from build123d import *

# Parameters (mm, degrees)
SKETCH_1_R      = 4
SKETCH_1_R_2    = 2
EXTRUDE_1_DEPTH = 2.8
SKETCH_1_3_R    = 2
EXTRUDE_2_DEPTH = 25
FILLET_1_R      = 0.5


with BuildPart() as part:
    # Sketch 1 → Extrude 1 (new body)
    # profile 1 of 2: a face of its own
    with BuildSketch(Plane(origin=(0, 0, 0), x_dir=(1, 0, 0), z_dir=(0, 1, 0))):
        with Locations(Location((0, 0, 0), (0, 0, 270))):
            Circle(SKETCH_1_R)
        Circle(SKETCH_1_R_2, mode=Mode.SUBTRACT)
    # profile 2 of 2: a face of its own
    with BuildSketch(Plane(origin=(0, 0, 0), x_dir=(1, 0, 0), z_dir=(0, 1, 0))):
        Circle(SKETCH_1_R_2)
    extrude(amount=EXTRUDE_1_DEPTH)

    # Sketch 1_3 → Extrude 2 (add)
    with BuildSketch(Plane(origin=(0, 0, 0), x_dir=(1, 0, 0), z_dir=(0, 1, 0))):
        with Locations(Location((0, 0, 0), (0, 0, 270))):
            Circle(SKETCH_1_3_R)
    extrude(amount=EXTRUDE_2_DEPTH)

    # Fillet 1
    fillet_1_edges = [part.edges().sort_by_distance(p)[0] for p in [
        (0, 0, -4),
    ]]
    fillet(fillet_1_edges, radius=FILLET_1_R)


solid = part.part
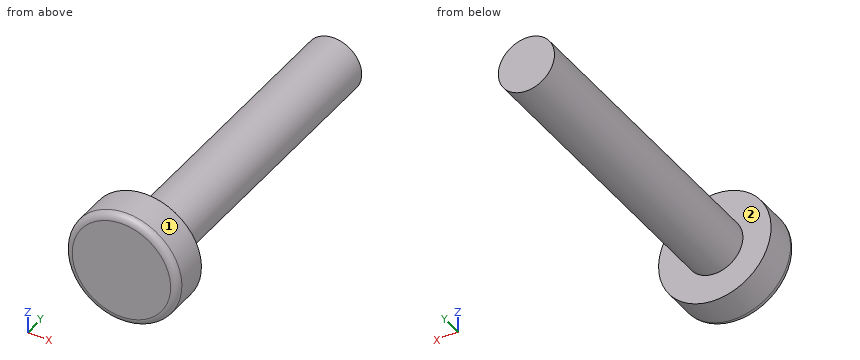
Build history of the part. All positions in model axes, mm. Face numbers are marked on the shaded views. A direction names the side the tool comes from. Round coordinates to 2 decimals unless told otherwise and drop trailing zeros. Write each loop counter-clockwise with the first axis right and the second up, starting at its lowest first coordinate (ties: lowest second). Pieces come first, ordered by that corner, then holes. Notation, with made-up numbers: M 29.5,-26.5 L 56.5,-26.5 A24 ccw 56.5,-0.5 Z; hole C 35.5,0 d7. An arc over 180 degrees is marked long. Use CSV: the item, a comma, the result in double quotes.
1. Tool access for the marked faces 1 and 2: list every direction of +Z, -Z, +X, -X, +Y, -Y with a clear straight run to the whole face (end or side of a thin tool).
Reply:
face 1,"+Y, -Y"
face 2,"+Y"
2. Saw through at B-B (z = 0). Give the cut face in (x, y), plus the area to 3 significant figures.
Reply:
outline,"M -4,0.5 A0.5 ccw -3.5,0 L 3.5,0 A0.5 ccw 4,0.5 L 4,2.8 L 2,2.8 L 2,25 L -2,25 L -2,2.8 L -4,2.8 Z"
area,"111 mm²"
3. Saw through at A-A (x = 0). Give the cut face in (y, z), plus the area to 3 significant figures.
Reply:
outline,"M 0,-3.5 A0.5 ccw 0.5,-4 L 2.8,-4 L 2.8,-2 L 25,-2 L 25,2 L 2.8,2 L 2.8,4 L 0.5,4 A0.5 ccw 0,3.5 Z"
area,"111 mm²"
4. Saw through at C-C (y = 23.25). Give the cut face in (x, z), plus the area to 3 significant figures.
Reply:
outline,"C 0,0 d4"
area,"12.6 mm²"
5. Flat gauge pins, fed straight in: pin 1 (3 mm diameter, centred on x = 0.5, y = 13.5, fed in from +Z); pin 2 (1 mm diameter, centred on x = 2.5, z = 0.5, fed in from +Y); pin 3 (1.5 mm diameter, centred on x = -2.5, y = 14, fed in from -Z). Where does each tip first touch, or does it go through?
Reply:
pin 1,"stops at z = 2"
pin 2,"stops at y = 2.8"
pin 3,"stops at z = -0.97"
6. Wall check: probe 1 along Y at (x, z) = (-2.75, 1.5); probe 2 along Z at (x, y) = (1.75, 12.75); probe 3 along Z at (x, y) = (1.5, 10). Give the ranges that are in metal, low to high. Write a range as from..to.
Reply:
probe 1,"y = 0..2.8"
probe 2,"z = -0.97..0.97"
probe 3,"z = -1.32..1.32"
